Geometry check sheet. Reference: the model listing, model coordinates, mm. A direction names the side the tool comes from. Coordinates: 2 decimals unless noted, no trailing zeros. Loops run counter-clockwise (first coordinate to the right, second up) from the corner with the lowest first, then second, coordinate; pieces in that order, holes last. Notation, with made-up numbers: (52.5, -24) - (70.5, -24) arc R8 ccw to (70.5, -15) - close; hole circle Ø3 at (6, 45). An arc over 180 degrees is marked (long way). One line per item, written item: value.
from build123d import *

# Parameters (mm, degrees)
SKETCH_R      = 42
PAD_DEPTH     = 2
SKETCH001_R   = 27.5
SKETCH001_R_2 = 20
PAD001_DEPTH  = 5
SKETCH002_R   = 22.5
SKETCH002_R_2 = 20
PAD002_DEPTH  = 10
CHAMFER_SIZE  = 1
SKETCH003_R   = 2
POCKET_DEPTH  = 2.001


with BuildPart() as part:
    # Sketch → Pad (new body)
    with BuildSketch(Plane.XY):
        Circle(SKETCH_R)
    extrude(amount=PAD_DEPTH)

    # Sketch001 (on Face3 of Pad) → Pad001 (join)
    with BuildSketch(Plane.XY.offset(2)):
        Circle(SKETCH001_R)
        Circle(SKETCH001_R_2, mode=Mode.SUBTRACT)
    extrude(amount=PAD001_DEPTH)

    # Sketch002 (on Face5 of Pad001) → Pad002 (join)
    with BuildSketch(Plane.XY.offset(7)):
        Circle(SKETCH002_R)
        Circle(SKETCH002_R_2, mode=Mode.SUBTRACT)
    extrude(amount=PAD002_DEPTH)

    # Chamfer
    chamfer_edges = [part.edges().sort_by_distance(p)[0] for p in [
        (-22.5, 0, 17),
    ]]
    chamfer(chamfer_edges, length=CHAMFER_SIZE)

    # Sketch003 (on Face10 of Chamfer) → Pocket (cut, through all)
    with BuildSketch(Plane.XY.offset(2)):
        with Locations((-10, 10)):
            Circle(SKETCH003_R)
        with Locations((10, 10)):
            Circle(SKETCH003_R)
        with Locations((10, -10)):
            Circle(SKETCH003_R)
        with Locations((-10, -10)):
            Circle(SKETCH003_R)
    extrude(amount=-POCKET_DEPTH, mode=Mode.SUBTRACT)


solid = part.part
(1) Cross-section at C-C on z = 12.5. Record the cut outline in (x, y).
Reply:
outline: circle Ø45 at (0, 0); hole circle Ø40 at (0, 0)
(2) Cross-section at A-A on x = 0. Record the cut outline in (y, z), and give its area (3 significant figures).
Reply:
outline: (-42, 0) - (42, 0) - (42, 2) - (27.5, 2) - (27.5, 7) - (22.5, 7) - (22.5, 16) - (21.5, 17) - (20, 17) - (20, 2) - (-20, 2) - (-20, 17) - (-21.5, 17) - (-22.5, 16) - (-22.5, 7) - (-27.5, 7) - (-27.5, 2) - (-42, 2) - close
area: 292 mm2
(3) Material ranges on probe 1 along Y at (x, z) = (-10, 0.5); probe 2 along Y at (x, z) = (0, 11.25); probe 3 along Z at (x, y) = (-3, 13), recorded low to high. Write a range as from..to.
Reply:
probe 1: -40.79..-12, -8..8, 12..40.79
probe 2: -22.5..-20, 20..22.5
probe 3: 0..2
(4) Release check for a two-part mould opening along X. For faces 3 (the face through (-5.961, -26.846, 4.465)), 4 (the face through (9, -27, 2)), 5 (the face through (-10, -8, 1)) record: pulls with the +X half, pulls with the -X half, needs draft (parallel to the pull), parting line crosses it, or undercut.
Reply:
face 3: parting line crosses it
face 4: needs draft
face 5: undercut
(5) Cross-section at D-D on y = -10. State how many separate pieces and enclosed holes the cut face has, and give its area (3 significant figures).
Reply:
separate pieces: 3
enclosed holes: 0
area: 286 mm2
(6) Access from +Z, -Z, +X, -X, +Y, -Y to the whole of each face (thin tool, end or side, straight path). Record for faces 1 (the face through (-10, 12, 1)), 2 (the face through (0, 0, 2)).
Reply:
face 1: +Z, -Z
face 2: +Z
(7) Go/stop test with flat-tipped pins: pin 1 Ø5 at (x, y) = (-10, 10) entering from +Z; pin 2 Ø3.5 at (x, y) = (10, -10) entering from +Z; pin 3 Ø2 at (y, z) = (-14, 12.5) entering from -X; pin 4 Ø6 at (y, z) = (26.5, 8) entering from -X. Record where each tip stops, or that it passes through.
Reply:
pin 1: z = 2
pin 2: through
pin 3: x = -18.36
pin 4: x = -14
